Part model, mm, in its own coordinate system. A direction names the side the tool comes from. Round coordinates to 2 decimals unless told otherwise and drop trailing zeros. Loops run counter-clockwise (first coordinate to the right, second up) from the corner with the lowest first, then second, coordinate; pieces in that order, holes last.
(1) Probe probe 1 along X at (y, z) = (92, 10.5); probe 2 along Z at (x, y) = (0, 98.7). List the from-to ranges inside material, lowest first.
(2) Flat gauge pins, fed straight in: pin 1 (1 mm diameter, centred on x = 7, z = -39.5, fed in from -Y); pin 2 (18 mm diameter, centred on x = -10, y = 35, fed in from -Z); pin 3 (5 mm diameter, centred on x = -28.5, y = 50.5, fed in from -Z). Where does each tip first touch, or does it go through?
(3) Tool access for faces 1 (the face through (-1, 50, -48)), 2 (the face through (0, 49, -50)), 3 (the face through (0, 49, 50)): list every direction of +Z, -Z, +X, -X, +Y, -Y with a clear straight run to the whole face (end or side of a thin tool).
(4) Cut at A-A on z = 0. List the corners of the cut face in (x, y), then the cut area to 3 significant figures.
(5) Cut at D-D on x = -40. List the corners of the cut face in (y, z), then the cut area to 3 significant figures.
(6) Mould opens along Z. For faces 4 (the face through (40, 49, -60)), 5 (the face through (-40, 49, 60)), 6 (the face through (-48, 50, 1)) say: +Z half, -Z half, draft (parallel to the pull), parting line (faces both ways), or undercut.
(7) Cut at C-C on y = 19.5. List the corners of the cut face in (x, z), then the cut area to 3 significant figures.
(8) Cut at B-B on x = 0. List the corners of the cut face in (y, z).
from build123d import *

# Parameters (mm, degrees)
SKETCH1_R           = 12.5
BOSS_EXTRUDE1_DEPTH = 100
SKETCH2_W           = 96
SKETCH2_H           = 96
CUT_EXTRUDE1_DEPTH  = 150


with BuildPart() as part:
    # Sketch1 → Boss-Extrude1 (new body)
    with BuildSketch(Plane(origin=(0, 0, 0), x_dir=(1, 0, 0), z_dir=(0, 1, 0))):
        with BuildLine():
            Line((-30, 50), (30, 50))
            ThreePointArc((30, 50), (40, 60), (50, 50))
            Line((50, 50), (50, -50))
            ThreePointArc((50, -50), (40, -60), (30, -50))
            Line((30, -50), (-30, -50))
            ThreePointArc((-30, -50), (-40, -60), (-50, -50))
            Line((-50, -50), (-50, 50))
            ThreePointArc((-50, 50), (-40, 60), (-30, 50))
        make_face()
        Circle(SKETCH1_R, mode=Mode.SUBTRACT)
    extrude(amount=BOSS_EXTRUDE1_DEPTH)

    # Sketch2 → Cut-Extrude1 (cut)
    with BuildSketch(Plane(origin=(0, 98, 0), x_dir=(1, 0, 0), z_dir=(0, 1, 0))):
        Rectangle(SKETCH2_W, SKETCH2_H)
    extrude(amount=-CUT_EXTRUDE1_DEPTH, mode=Mode.SUBTRACT)


solid = part.part
Final values:
1. probe 1: x = -50 to -48, 48 to 50
1. probe 2: z = -50 to -12.5, 12.5 to 50
2. pin 1: stops at y = 98
2. pin 2: stops at z = -50
2. pin 3: stops at z = -54.36
3. face 1: -Y
3. face 2: -Z, +Y, -Y
3. face 3: +Z, +Y, -Y
4. outline: (-50, 0) - (-48, 0) - (-48, 98) - (-12.5, 98) - (-12.5, 100) - (-50, 100) - close; (12.5, 98) - (48, 98) - (48, 0) - (50, 0) - (50, 100) - (12.5, 100) - close
4. area: 542 mm2
5. outline: (0, -60) - (100, -60) - (100, 60) - (0, 60) - (0, 48) - (98, 48) - (98, -48) - (0, -48) - close
5. area: 2,590 mm2
6. face 4: -Z half
6. face 5: +Z half
6. face 6: undercut
7. outline: (-50, -50) arc R10 ccw to (-30, -50) - (30, -50) arc R10 ccw to (50, -50) - (50, 50) arc R10 ccw to (30, 50) - (-30, 50) arc R10 ccw to (-50, 50) - close; hole (-48, -48) - (48, -48) - (48, 48) - (-48, 48) - close
7. area: 1,410 mm2
8. outline: (0, -50) - (100, -50) - (100, -12.5) - (98, -12.5) - (98, -48) - (0, -48) - close; (0, 48) - (98, 48) - (98, 12.5) - (100, 12.5) - (100, 50) - (0, 50) - close
